Build history of the part. All positions in model axes, mm. Face numbers are marked on the shaded views. Coordinates: 2 decimals unless noted, no trailing zeros. Loops run counter-clockwise (first coordinate to the right, second up) from the corner with the lowest first, then second, coordinate; pieces in that order, holes last.
Item 1: Cut at A-A (z = 16.75). List the corners of the cut face in (x, y).
Item 2: Flat gauge pins, fed straight in: pin 1 (5 mm diameter, centred on x = 0, z = 6, fed in from -Y); pin 2 (4 mm diameter, centred on y = -9.5, z = 4.5, fed in from +X); pin 3 (1 mm diameter, centred on y = 7, z = 7, fed in from -X). Where does each tip first touch, or does it go through?
Item 3: Drill centre lines: line 1 along Y through (x, z) = (0, 6); line 2 along Z through (x, y) = (-14, -2); line 3 along Y through (x, z) = (-9, 6.25). Where is each one in solid material? Low to high.
Item 4: Mould opens along Y. For the marked faces 1, 2, 3 and 4 say: released by +Y, released by -Y, zero draft, split by the parting line, or undercut.
Item 5: Cut at B-B (x = 0). List the corners of the cut face in (y, z), and give its area (3 significant figures).
from build123d import *

# Parameters (mm, degrees)
SKETCH1_R           = 22.75
BOSS_EXTRUDE1_DEPTH = 2
SKETCH2_R           = 22.675423682
SKETCH2_R_2         = 20.675423682
BOSS_EXTRUDE2_DEPTH = 20
FILLET1_R           = 1


with BuildPart() as part:
    # Sketch1 → Boss-Extrude1 (new body)
    with BuildSketch(Plane.XY):
        Circle(SKETCH1_R)
    extrude(amount=BOSS_EXTRUDE1_DEPTH)

    # Sketch2 → Boss-Extrude2 (add)
    with BuildSketch(Plane.XY.offset(2)):
        Circle(SKETCH2_R)
        Circle(SKETCH2_R_2, mode=Mode.SUBTRACT)
    extrude(amount=BOSS_EXTRUDE2_DEPTH)

    # Fillet1
    fillet1_edges = [part.edges().sort_by_distance(p)[0] for p in [
        (-22.75, 0, 0),
    ]]
    fillet(fillet1_edges, radius=FILLET1_R)


solid = part.part
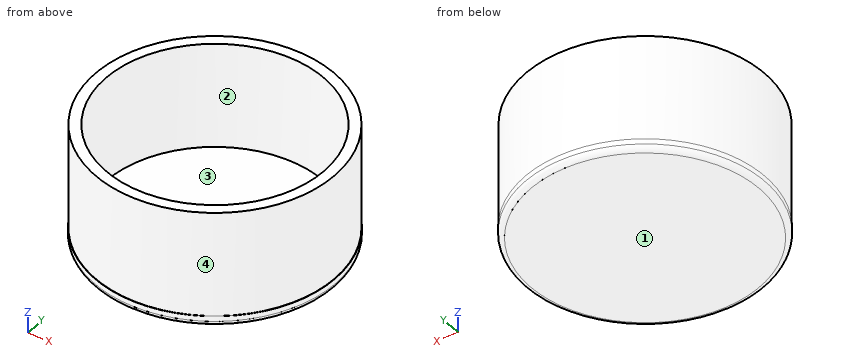
Filled sheet:
1. outline: circle Ø45.35 at (0, 0); hole circle Ø41.35 at (0, 0)
2. pin 1: stops at y = -22.68
2. pin 2: stops at x = 21.4
2. pin 3: stops at x = -21.72
3. line 1: y = -22.68 to -20.68, 20.68 to 22.68
3. line 2: z = 0 to 2
3. line 3: y = -20.81 to -18.61, 18.61 to 20.81
4. face 1: zero draft
4. face 2: undercut
4. face 3: undercut
4. face 4: split by the parting line
5. outline: (-22.75, 1) arc R1 ccw to (-21.75, 0) - (21.75, 0) arc R1 ccw to (22.75, 1) - (22.75, 2) - (22.68, 2) - (22.68, 22) - (20.68, 22) - (20.68, 2) - (-20.68, 2) - (-20.68, 22) - (-22.68, 22) - (-22.68, 2) - (-22.75, 2) - close
5. area: 171 mm2
